Part model, mm, in its own coordinate system. A direction names the side the tool comes from. Round coordinates to 2 decimals unless told otherwise and drop trailing zeros. Order: outer loops, then holes, each group sorted by start corner. A loop starts at its lowest first (then second) coordinate and runs counter-clockwise, first axis right, second up. Notation, with made-up numbers: (67, 72.25) - (75, 72.25) arc R26 cw to (75, 97.25) - close; hole circle Ø6 at (75, 61). An arc over 180 degrees is marked (long way). Answer as a JSON object with one key per item and string values.
Autodesk Inventor part; units mm, degrees
ref_plane "Work Plane3" through (167.8, -16.921, -48) normal (-1, 0, 0) x (0, 0, 1)
ref_plane "YZ Plane" through (0, 0, 0) normal (1, 0, 0) x (0, 1, 0)
ref_plane "XZ Plane" through (0, 0, 0) normal (0, 1, 0) x (-1, 0, 0)
ref_plane "Work Plane1" through (182.8, -16.921, -7.958) normal (0, -1, 0) x (0, 0, -1)
ref_plane "Work Plane2" through (182.8, -6.9868, -42.1222) normal (1, 0, 0) x (0, 0, -1)
sketch "Sketch1" plane through (182.8, -6.9868, -42.1222) normal (1, 0, 0) x (0, 0, -1)
  arc A0 (5.0194, 6.9868) -> (5.8778, 5.8182) centre (7.8778, 8.1868) ccw
  line L0 (-9.7772, 6.9868) -> (5.0194, 6.9868)
  arc A1 (-7.9865, 5.8774) -> (-9.7772, 6.9868) centre (-9.7772, 4.9868) ccw
  line L1 (-7.9865, 5.8774) -> (-0.1222, -9.9342)
  line L2 (-0.1222, -9.9342) -> (5.8778, -9.9342)
  line L3 (5.8778, -9.9342) -> (5.8778, 5.8182)
  line L4 (-42.1222, 6.9868) -> (-42.1222, -9.9342)
  line L5 (-42.1222, -9.9342) -> (-34.1642, -9.9342)
  line L6 (-34.1642, -9.9342) -> (-26.2998, 5.8774)
  arc A2 (-24.5091, 6.9868) -> (-26.2998, 5.8774) centre (-24.5091, 4.9868) ccw
  line L7 (-42.1222, 6.9868) -> (-24.5091, 6.9868)
  circle A3 centre (-17.1432, -9.9342) radius 15.24 construction
  line L8 (-17.1432, -9.9342) -> (-17.1432, -20.9232) construction
  line L9 (-17.1432, -9.9342) -> (-6.1542, -9.9342) construction
  line L10 (-0.1222, -9.9342) -> (-8.2255, -25.1742)
  line L11 (-0.1222, -9.9342) -> (17.1381, -9.9342) construction
  line L12 (-8.2255, -25.1742) -> (-17.1432, -25.1742)
  line L13 (-17.1432, -25.1742) -> (-17.1432, -28.1742)
  line L14 (-17.1432, -28.1742) -> (5.8778, -28.1742)
  line L15 (5.8778, -28.1742) -> (5.8778, -9.9342)
  line L16 (-0.1222, -9.9342) -> (5.8778, -9.9342)
  dimension "d0" = 90
  dimension "d1" = 118
  dimension "d2" = 3
  dimension "d3" = 90
ref_plane "Work Plane3" through (167.8, -16.921, -48) normal (-1, 0, 0) x (0, 0, 1)
extrude "Extrusion1" add sketch "Sketch1" against normal up to surface (15 mm away) contours L15 L14 L13 L12 L10 L2
sketch "Sketch2" plane through (182.8, -35.161, -48) normal (0, -1, 0) x (1, 0, 0)
  circle A0 centre (-7.5, 3) radius 1.45
  point P0 (-182.8, 48)
hole "Hole1" at (175.3, -35.161, -45) direction (0, 1, 0) diameter 3.5 end through all counterbore diameter 6 counterbore depth 6.5
mirror "Mirror1" about plane through (182.8, -35.161, -24.979) normal (0, 0, 1) of "Extrusion1", "Hole1"
properties part number "30_CUBE_openSIM_Lensfixation"
Item 1: Cut at D-D (x = 175.75). State how many separate pieces and enclosed holes the cut face has, plus the area to 3 significant figures.
Taken from the geometry:
{"separate pieces": "3", "enclosed holes": "0", "area": "288 mm2"}
Item 2: Cut at C-C (x = 180.25). Write the cut outline in (y, z).
Taken from the geometry:
{"outline": "(-35.16, -48) - (-16.92, -48) - (-16.92, -42) - (-32.16, -33.9) - (-32.16, -16.06) - (-16.92, -7.96) - (-16.92, -1.96) - (-35.16, -1.96) - close"}
Item 3: Cut at A-A (y = -21.75). Write the cut outline in (x, z).
Taken from the geometry:
{"outline": "(167.8, -48) - (182.8, -48) - (182.8, -39.43) - (167.8, -39.43) - close; (167.8, -10.53) - (182.8, -10.53) - (182.8, -1.96) - (167.8, -1.96) - close; hole circle Ø3.5 at (175.3, -45); hole circle Ø3.5 at (175.3, -4.96)"}
Item 4: Cut at B-B (z = -45). Write the cut outline in (x, y), plus the area to 3 significant figures.
Taken from the geometry:
{"outline": "(167.8, -35.16) - (172.3, -35.16) - (172.3, -28.66) - (173.55, -28.66) - (173.55, -16.92) - (167.8, -16.92) - close; (177.05, -28.66) - (178.3, -28.66) - (178.3, -35.16) - (182.8, -35.16) - (182.8, -16.92) - (177.05, -16.92) - close", "area": "194 mm2"}
Item 5: Drop flat-ended pins along their axis: P1, Ø3, axis at x = 175.3, z = -4.958, coming from the +Y side; P2, Ø6, axis at x = 175.5, z = -15, coming from the +Y side; P3, Ø5.5, axis at x = 175.3, z = -45, coming from the -Y side; P4, Ø8, axis at x = 178.5, z = -33, coming from the +Y side. Give the stop position or say it passes through.
Taken from the geometry:
{"P1": "through", "P2": "y = -24.52", "P3": "y = -28.66", "P4": "y = -26.32"}
Item 6: Two-plate mould, pull along X, no slides. Class faces 1 (the flat face through (182.8, -34, -25)), 2 (the flat face through (177, -28.661, -6)), 3 (the flat face through (175.405, -24.434, -38.005)): pulls with the +X half, pulls with the -X half, needs draft (parallel to the pull), parting line crosses it, or undercut.
Taken from the geometry:
{"face 1": "pulls with the +X half", "face 2": "undercut", "face 3": "needs draft"}
Item 7: Tool access for faces 4 (the flat face through (175.405, -24.648, -12.066)), 5 (the cylindrical face through (176.85, -22.71, -45.81)), 6 (the cylindrical face through (177.8, -31.9, -3.3)): list every direction of +Z, -Z, +X, -X, +Y, -Y with a clear straight run to the whole face (end or side of a thin tool).
Taken from the geometry:
{"face 4": "+X, -X, +Y", "face 5": "+Y, -Y", "face 6": "-Y"}
Item 8: Probe L1, parallel to Z at x = 175.3, y = -24.25; L2, parallel to Z at x = 175.3, y = -22.25; L3, parallel to X at y = -24.75, z = -45. List the from-to ranges inside material, lowest first. Write a range as from..to.
Taken from the geometry:
{"L1": "-48..-46.75, -43.25..-38.1, -11.85..-6.71, -3.21..-1.96", "L2": "-48..-46.75, -43.25..-39.17, -10.79..-6.71, -3.21..-1.96", "L3": "167.8..173.55, 177.05..182.8"}
